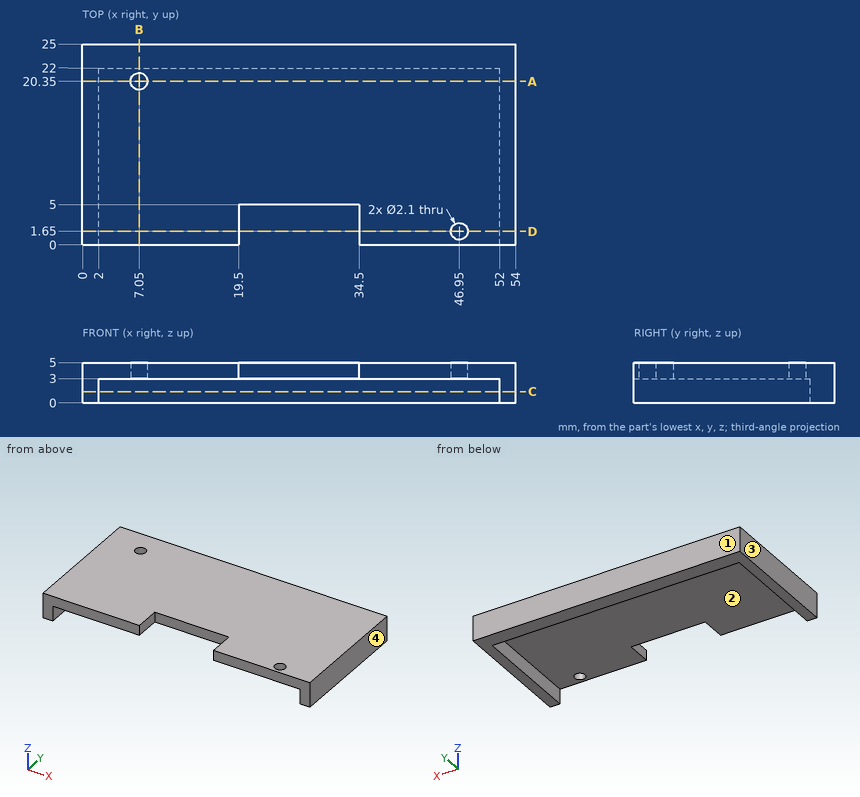
Input: dimensioned drawing with shaded views. Units: mm. Origin: part minimum x, y, z. Coordinates: 2 decimals unless noted, no trailing zeros. Loops run counter-clockwise (first coordinate to the right, second up) from the corner with the lowest first, then second, coordinate; pieces in that order, holes last. Notation, with made-up numbers: M 30,2 L 78,2 A18 ccw 78,12 Z; hole C 68.25,-15.75 d11. An arc over 180 degrees is marked long. One line per item, written item: value. Start each with the question number.
1) Cut plane C-C (z = 1.4). Return loops of the section in (x, y), then the cut area to 3 significant figures.
2) Cut plane A-A (y = 20.35). Return loops of the section in (x, z).
3) Draft query along X for the marked faces 1, 2, 3 and 4. Return one class per face: released by +X, released by -X, zero draft, split by the parting line, or undercut.
4) Material intervals for L1, parallel to Y at x = 7.05, z = 3.4; L2, parallel to Y at x = 46.95, z = 3.7; L3, parallel to Z at x = 23, y = 14.75, sorted ascending. Write a range as from..to.
5) Cut plane D-D (y = 1.65). Return loops of the section in (x, z).
6) Pin query (flat end, axial travel): P1, Ø1, axis at x = 9, y = 4.5, coming from the -Z side; P2, Ø1.6, axis at x = 24, z = 4, coming from the -Y side; P3, Ø1.5, axis at x = 32.5, z = 1.5, coming from the -Y side. Return the tip coordinate at first contact, or that it passes through.
7) Cut plane B-B (x = 7.05). Return loops of the section in (y, z), then the cut area to 3 significant figures.
Evaluation:
1. outline: M 0,0 L 2,0 L 2,22 L 52,22 L 52,0 L 54,0 L 54,25 L 0,25 Z
1. area: 250 mm^2
2. outline: M 0,0 L 2,0 L 2,3 L 6,3 L 6,5 L 0,5 Z; M 8.1,3 L 52,3 L 52,0 L 54,0 L 54,5 L 8.1,5 Z
3. face 1: zero draft
3. face 2: undercut
3. face 3: released by -X
3. face 4: released by +X
4. L1: 0..19.3, 21.4..25
4. L2: 0..0.6, 2.7..25
4. L3: 3..5
5. outline: M 0,0 L 2,0 L 2,3 L 19.5,3 L 19.5,5 L 0,5 Z; M 34.5,3 L 45.9,3 L 45.9,5 L 34.5,5 Z; M 48,3 L 52,3 L 52,0 L 54,0 L 54,5 L 48,5 Z
6. P1: z = 3
6. P2: y = 5
6. P3: y = 22
7. outline: M 0,3 L 19.3,3 L 19.3,5 L 0,5 Z; M 21.4,3 L 22,3 L 22,0 L 25,0 L 25,5 L 21.4,5 Z
7. area: 54.8 mm^2
